Autodesk Inventor part; units mm, degrees
ref_plane "side_4d_XY" through (-20, 0, -350) normal (-1, 0, 0) x (0, 1, 0)
ref_plane "side_4d_YZ" through (-20, 0, -350) normal (0, 1, 0) x (0, 0, -1)
ref_plane "side_4d_ZX" through (-20, 0, -350) normal (0, 0, -1) x (-1, 0, 0)
sketch "Skizze_1" plane through (0, 0, 0) normal (0, 0, 1) x (1, 0, 0)
  arc A0 (-20, -17) -> (-17, -20) centre (-17, -17) ccw
  line L0 (-17, -20) -> (-4.1, -20)
  line L1 (-4.1, -20) -> (-4.1, -17)
  line L2 (-4.1, -17) -> (-10.5, -17)
  line L3 (-10.5, -17) -> (-10.5, -13.6627)
  arc A1 (-10.0314, -12.5314) -> (-10.5, -13.6627) centre (-8.9002, -13.6627) ccw
  line L4 (-10.0314, -12.5314) -> (-7.4645, -9.9645)
  arc A2 (-3.9289, -8.5) -> (-7.4645, -9.9645) centre (-3.9289, -13.5) ccw
  line L5 (-3.9289, -8.5) -> (3.9289, -8.5)
  arc A3 (7.4645, -9.9645) -> (3.9289, -8.5) centre (3.9289, -13.5) ccw
  line L6 (7.4645, -9.9645) -> (10.0314, -12.5314)
  arc A4 (10.5, -13.6627) -> (10.0314, -12.5314) centre (8.9002, -13.6627) ccw
  line L7 (10.5, -13.6627) -> (10.5, -17)
  line L8 (10.5, -17) -> (4.1, -17)
  line L9 (4.1, -17) -> (4.1, -20)
  line L10 (4.1, -20) -> (17, -20)
  arc A5 (17, -20) -> (20, -17) centre (17, -17) ccw
  line L11 (20, -17) -> (20, -4.1)
  line L12 (20, -4.1) -> (17, -4.1)
  line L13 (17, -4.1) -> (17, -10.5)
  line L14 (17, -10.5) -> (13.6627, -10.5)
  arc A6 (12.5314, -10.0314) -> (13.6627, -10.5) centre (13.6627, -8.9002) ccw
  line L15 (12.5314, -10.0314) -> (9.9645, -7.4645)
  arc A7 (8.5, -3.9289) -> (9.9645, -7.4645) centre (13.5, -3.9289) ccw
  line L16 (8.5, -3.9289) -> (8.5, 3.9289)
  arc A8 (9.9645, 7.4645) -> (8.5, 3.9289) centre (13.5, 3.9289) ccw
  line L17 (9.9645, 7.4645) -> (12.5314, 10.0314)
  arc A9 (13.6627, 10.5) -> (12.5314, 10.0314) centre (13.6627, 8.9002) ccw
  line L18 (13.6627, 10.5) -> (17, 10.5)
  line L19 (17, 10.5) -> (17, 4.1)
  line L20 (17, 4.1) -> (20, 4.1)
  line L21 (20, 4.1) -> (20, 17)
  arc A10 (20, 17) -> (17, 20) centre (17, 17) ccw
  line L22 (17, 20) -> (4.1, 20)
  line L23 (4.1, 20) -> (4.1, 17)
  line L24 (4.1, 17) -> (10.5, 17)
  line L25 (10.5, 17) -> (10.5, 13.6627)
  arc A11 (10.0314, 12.5314) -> (10.5, 13.6627) centre (8.9002, 13.6627) ccw
  line L26 (10.0314, 12.5314) -> (7.4645, 9.9645)
  arc A12 (3.9289, 8.5) -> (7.4645, 9.9645) centre (3.9289, 13.5) ccw
  line L27 (3.9289, 8.5) -> (-3.9289, 8.5)
  arc A13 (-7.4645, 9.9645) -> (-3.9289, 8.5) centre (-3.9289, 13.5) ccw
  line L28 (-7.4645, 9.9645) -> (-10.0314, 12.5314)
  arc A14 (-10.5, 13.6627) -> (-10.0314, 12.5314) centre (-8.9002, 13.6627) ccw
  line L29 (-10.5, 13.6627) -> (-10.5, 17)
  line L30 (-10.5, 17) -> (-4.1, 17)
  line L31 (-4.1, 17) -> (-4.1, 20)
  line L32 (-4.1, 20) -> (-17, 20)
  arc A15 (-17, 20) -> (-20, 17) centre (-17, 17) ccw
  line L33 (-20, 17) -> (-20, 4.1)
  line L34 (-20, 4.1) -> (-17, 4.1)
  line L35 (-17, 4.1) -> (-17, 10.5)
  line L36 (-17, 10.5) -> (-13.6627, 10.5)
  arc A16 (-12.5314, 10.0314) -> (-13.6627, 10.5) centre (-13.6627, 8.9002) ccw
  line L37 (-12.5314, 10.0314) -> (-9.9645, 7.4645)
  arc A17 (-8.5, 3.9289) -> (-9.9645, 7.4645) centre (-13.5, 3.9289) ccw
  line L38 (-8.5, 3.9289) -> (-8.5, -3.9289)
  arc A18 (-9.9645, -7.4645) -> (-8.5, -3.9289) centre (-13.5, -3.9289) ccw
  line L39 (-9.9645, -7.4645) -> (-12.5314, -10.0314)
  arc A19 (-13.6627, -10.5) -> (-12.5314, -10.0314) centre (-13.6627, -8.9002) ccw
  line L40 (-13.6627, -10.5) -> (-17, -10.5)
  line L41 (-17, -10.5) -> (-17, -4.1)
  line L42 (-17, -4.1) -> (-20, -4.1)
  line L43 (-20, -4.1) -> (-20, -17)
  circle A20 centre (0, 0) radius 6
extrude "Extrusion1" add sketch "Skizze_1" against normal blind 700
sketch "Sketch2" plane through (0, 0, 0) normal (0, 0, 1) x (1, 0, 0)
  point P0 (-15, -15)
hole "Drilling 1" at (-15, -15, 0) direction (0, 0, -1) diameter 5 depth 6000
sketch "Sketch3" plane through (0, 0, 0) normal (0, 0, 1) x (1, 0, 0)
  point P0 (15, -15)
hole "Drilling 2" at (15, -15, 0) direction (0, 0, -1) diameter 5 depth 6000
sketch "Sketch4" plane through (0, 0, 0) normal (0, 0, 1) x (1, 0, 0)
  point P0 (15, 15)
hole "Drilling 3" at (15, 15, 0) direction (0, 0, -1) diameter 5 depth 6000
sketch "Sketch5" plane through (0, 0, 0) normal (0, 0, 1) x (1, 0, 0)
  point P0 (-15, 15)
hole "Drilling 4" at (-15, 15, 0) direction (0, 0, -1) diameter 5 depth 6000
ref_plane "side_4d_XY" through (-20, 0, -350) normal (-1, 0, 0) x (0, 1, 0)
ref_plane "side_4d_YZ" through (-20, 0, -350) normal (0, 1, 0) x (0, 0, -1)
ref_plane "side_4d_ZX" through (-20, 0, -350) normal (0, 0, -1) x (-1, 0, 0)
ref_plane "side_1a_XY" through (0, 20, -350) normal (0, 1, 0) x (1, 0, 0)
ref_plane "side_1a_YZ" through (0, 20, -350) normal (1, 0, 0) x (0, 0, -1)
ref_plane "side_1a_ZX" through (0, 20, -350) normal (0, 0, -1) x (0, 1, 0)
ref_plane "side_2b_XY" through (20, 0, -350) normal (1, 0, 0) x (0, -1, 0)
ref_plane "side_2b_YZ" through (20, 0, -350) normal (0, -1, 0) x (0, 0, -1)
ref_plane "side_2b_ZX" through (20, 0, -350) normal (0, 0, -1) x (1, 0, 0)
ref_plane "side_3c_XY" through (0, -20, -350) normal (0, -1, 0) x (-1, 0, 0)
ref_plane "side_3c_YZ" through (0, -20, -350) normal (-1, 0, 0) x (0, 0, -1)
ref_plane "side_3c_ZX" through (0, -20, -350) normal (0, 0, -1) x (0, -1, 0)
ref_plane "end_XY" through (0, 0, -700) normal (0, 0, -1) x (1, 0, 0)
ref_plane "end_YZ" through (0, 0, -700) normal (1, 0, 0) x (0, -1, 0)
ref_plane "end_ZX" through (0, 0, -700) normal (0, -1, 0) x (0, 0, -1)
ref_plane "start_XY" through (0, 0, 0) normal (0, 0, 1) x (1, 0, 0)
ref_plane "start_YZ" through (0, 0, 0) normal (1, 0, 0) x (0, 1, 0)
ref_plane "start_ZX" through (0, 0, 0) normal (0, 1, 0) x (0, 0, 1)
properties part number "MayTec 1.11.040040.43S_Profile 40x40, 4E, S_700_Detail_(0;0,0,0)"
Build history of the part. All positions in model axes, mm. Give positions to 0.01 mm unless a question says otherwise; leave off trailing zeros.
Item 1: Drill centre lines: line 1 (X direction, y = -15, z = -532); line 2 (Y direction, x = 10, z = -271). Where is each one in solid material? Low to high.
Answers follow:
line 1: x = -20 to -17.5, -12.5 to -10.5, 10.5 to 12.5, 17.5 to 20
line 2: y = -20 to -17, -12.5 to -7.5, 7.5 to 12.5, 17 to 20
Item 2: Pull direction Y, two halves, no side cores. Call faces 1 (the face through (-10, 20, -345)), 2 (the face through (-5, -4, -700)), 3 (the face through (-6, 0, -345)): released by +Y, released by -Y, zero draft, split by the parting line, or undercut.
Answers follow:
face 1: released by +Y
face 2: zero draft
face 3: undercut
Item 3: Flat gauge pin, fed straight in: pin 1 (1 mm diameter, centred on x = 3.5, z = -203, fed in from +Y). Where does the tip first touch, or does it go through?
Answers follow:
pin 1: stops at y = 8.5
Item 4: Slice it at A-A, the plane z = -264. Give the number of separate pieces and of enclosed holes in the cut face, and give its area (3 significant figures).
Answers follow:
separate pieces: 1
enclosed holes: 5
area: 674 mm2
